from build123d import *

# Parameters (mm, degrees)
IZIM1_W                     = 35
IZIM1_H                     = 35
IZIM1_W_2                   = 29
IZIM1_H_2                   = 29
Y_KSEKLIK_EKSTR_ZYON1_DEPTH = 35
IZIM2_W                     = 35
IZIM2_H                     = 35
Y_KSEKLIK_EKSTR_ZYON2_DEPTH = 2.5
IZIM7_R                     = 1.25
KES_EKSTR_ZYON5_DEPTH       = 75.246212025
IZIM5_R                     = 9.125
KES_EKSTR_ZYON3_DEPTH       = 72.894019223
IZIM10_W                    = 50
IZIM10_H                    = 50
IZIM10_W_2                  = 30.1
IZIM10_H_2                  = 30.1
Y_KSEKLIK_EKSTR_ZYON3_DEPTH = 75
IZIM12_W                    = 50
IZIM12_H                    = 50
IZIM12_W_2                  = 35
IZIM12_H_2                  = 35
Y_KSEKLIK_EKSTR_ZYON4_DEPTH = 20
KES_EKSTR_ZYON1_DEPTH       = 121.545634512
KES_EKSTR_ZYON6_START       = -10
KES_EKSTR_ZYON6_DEPTH       = 10
DAIRESEL_KAPLAMA1_COUNT     = 4
KES_EKSTR_ZYON7_DEPTH       = 124.389626793
KES_EKSTR_ZYON8_DEPTH       = 124.389626793
RADYUS4_R                   = 10
KES_EKSTR_ZYON9_DEPTH       = 121.545634512


with BuildPart() as part:
    # izim1 → Y_kseklik-Ekstr_zyon1 (new, symmetric)
    with BuildSketch(Plane.XY):
        Rectangle(IZIM1_W, IZIM1_H)
        Rectangle(IZIM1_W_2, IZIM1_H_2, mode=Mode.SUBTRACT)
    extrude(amount=Y_KSEKLIK_EKSTR_ZYON1_DEPTH, both=True)

    # izim2 → Y_kseklik-Ekstr_zyon2 (add)
    with BuildSketch(Plane.XY.offset(35)):
        Rectangle(IZIM2_W, IZIM2_H)
    extrude(amount=-Y_KSEKLIK_EKSTR_ZYON2_DEPTH)

    # izim7 → Kes-Ekstr_zyon5 (cut, through all)
    with BuildSketch(Plane.XY.offset(35)):
        with Locations((-11, 0)):
            Circle(IZIM7_R)
        with Locations((11, 0)):
            Circle(IZIM7_R)
        with Locations((0, 11)):
            Circle(IZIM7_R)
        with Locations((0, -11)):
            Circle(IZIM7_R)
    extrude(amount=-KES_EKSTR_ZYON5_DEPTH, mode=Mode.SUBTRACT)

    # izim5 → Kes-Ekstr_zyon3 (cut, through all)
    with BuildSketch(Plane(origin=(0, 0, 32.5), x_dir=(-1, 0, 0), z_dir=(0, 0, -1))):
        Circle(IZIM5_R)
    extrude(amount=-KES_EKSTR_ZYON3_DEPTH, mode=Mode.SUBTRACT)



with BuildPart() as body_2:
    # izim10 → Y_kseklik-Ekstr_zyon3 (new body)
    with BuildSketch(Plane(origin=(0, 0, -35), x_dir=(-1, 0, 0), z_dir=(0, 0, -1))):
        Rectangle(IZIM10_W, IZIM10_H)
        Rectangle(IZIM10_W_2, IZIM10_H_2, mode=Mode.SUBTRACT)
    extrude(amount=Y_KSEKLIK_EKSTR_ZYON3_DEPTH)


with BuildPart() as part_1:
    add(part.part)

    add(body_2.part)  # Y_kseklik-Ekstr_zyon4 merges body 2
    # izim12 → Y_kseklik-Ekstr_zyon4 (add)
    with BuildSketch(Plane.XY.offset(-35)):
        Rectangle(IZIM12_W, IZIM12_H)
        Rectangle(IZIM12_W_2, IZIM12_H_2, mode=Mode.SUBTRACT)
    extrude(amount=Y_KSEKLIK_EKSTR_ZYON4_DEPTH)

    # izim3 → Kes-Ekstr_zyon1 (cut, through all)
    with BuildSketch(Plane(origin=(0, 17.5, 0), x_dir=(1, 0, 0), z_dir=(0, 1, 0))):
        with BuildLine():
            Line((10, 20), (10, -20))
            ThreePointArc((10, -20), (0, -30), (-10, -20))
            Line((-10, -20), (-10, 20))
            ThreePointArc((-10, 20), (0, 30), (10, 20))
        make_face()
    kes_ekstr_zyon1 = extrude(amount=-KES_EKSTR_ZYON1_DEPTH, mode=Mode.SUBTRACT)

    # izim8 → Kes-Ekstr_zyon6 (cut)
    with BuildSketch(Plane.XZ.offset(17.5).offset(KES_EKSTR_ZYON6_START)):
        with BuildLine():
            Line((-10, -20), (-10, -35))
            Line((-10, -35), (10, -35))
            Line((10, -35), (10, -20))
            ThreePointArc((10, -20), (0, -30), (-10, -20))
        make_face()
    extrude(amount=KES_EKSTR_ZYON6_DEPTH, mode=Mode.SUBTRACT)

    # Dairesel Kaplama1: Kes-Ekstr_zyon1 ×4 about axis
    dairesel_kaplama1_axis = Axis((0, 0, 0), (0, 0, 1))
    for i in range(1, DAIRESEL_KAPLAMA1_COUNT):
        add(kes_ekstr_zyon1.rotate(dairesel_kaplama1_axis, i * 360 / DAIRESEL_KAPLAMA1_COUNT), mode=Mode.SUBTRACT)

    # izim13 → Kes-Ekstr_zyon7 (cut, through all)
    with BuildSketch(Plane(origin=(25, 0, 0), x_dir=(0, 0, -1), z_dir=(1, 0, 0))):
        Polygon((15, 25), (15, 17.5), (35, 25), align=None)
        Polygon((15, -17.5), (15, -25), (35, -25), align=None)
    extrude(amount=-KES_EKSTR_ZYON7_DEPTH, mode=Mode.SUBTRACT)

    # izim14 → Kes-Ekstr_zyon8 (cut, through all)
    with BuildSketch(Plane.XZ.offset(25)):
        Polygon((-17.5, -15), (-25, -35), (-25, -15), align=None)
        Polygon((17.5, -15), (25, -15), (25, -35), align=None)
    extrude(amount=-KES_EKSTR_ZYON8_DEPTH, mode=Mode.SUBTRACT)

    # Radyus4
    # the kernel refuses this fillet: 10 mm, written as the material it takes off along each edge
    with BuildSketch(Plane(origin=(32.317073171, 32.317073171, -54.512195122), x_dir=(-0.9435273723846194, 0.11632529248577513, -0.31020077996206696), z_dir=(-0.33129457822453995, -0.3312945782245377, 0.883452208598773))) as radyus4_piece_1_section:
        with BuildLine():
            CenterArc((RADYUS4_R * 0.883452208599, RADYUS4_R), RADYUS4_R, 187.08188169, 82.91811831)
            Line((-RADYUS4_R * 0.108918765444, RADYUS4_R * 0.876712328767), (0, 0))
            Line((0, 0), (RADYUS4_R * 0.883452208599, 0))
        make_face()
    radyus4_piece_1 = extrude(amount=66.811073275, mode=Mode.PRIVATE)
    radyus4_piece_1 = split(radyus4_piece_1, bisect_by=Plane(origin=(17.5, 21.25, -29.89398757), z_dir=(1, 0, 0)), keep=Keep.TOP, mode=Mode.PRIVATE)
    add(radyus4_piece_1, mode=Mode.SUBTRACT)
    with BuildSketch(Plane(origin=(32.317073171, 32.317073171, -54.512195122), x_dir=(-0.9435273723846194, 0.11632529248577513, -0.31020077996206696), z_dir=(-0.33129457822453995, -0.3312945782245377, 0.883452208598773))) as radyus4_piece_2_section:
        with BuildLine():
            CenterArc((RADYUS4_R * 0.883452208599, RADYUS4_R), RADYUS4_R, 187.08188169, 82.91811831)
            Line((-RADYUS4_R * 0.108918765444, RADYUS4_R * 0.876712328767), (0, 0))
            Line((0, 0), (RADYUS4_R * 0.883452208599, 0))
        make_face()
    radyus4_piece_2 = extrude(amount=66.811073275, mode=Mode.PRIVATE)
    radyus4_piece_2 = split(radyus4_piece_2, bisect_by=Plane(origin=(16.256655696, 17.5, -22.379324277), z_dir=(0, 1, 0)), keep=Keep.TOP, mode=Mode.PRIVATE)
    add(radyus4_piece_2, mode=Mode.SUBTRACT)
    with BuildSketch(Plane(origin=(-10.182926829, 10.182926829, 4.512195122), x_dir=(0.943527372384614, 0.11632529248577986, -0.3102007799620813), z_dir=(-0.33129457822455505, 0.3312945782245359, -0.883452208598768))) as radyus4_piece_3_section:
        with BuildLine():
            CenterArc((RADYUS4_R * 0.883452208599, RADYUS4_R), RADYUS4_R, 187.08188169, 82.91811831)
            Line((-RADYUS4_R * 0.108918765444, RADYUS4_R * 0.876712328767), (0, 0))
            Line((0, 0), (RADYUS4_R * 0.883452208599, 0))
        make_face()
    radyus4_piece_3 = extrude(amount=66.811073275, mode=Mode.PRIVATE)
    radyus4_piece_3 = split(radyus4_piece_3, bisect_by=Plane(origin=(-17.5, 13.216664443, -19.287647888), z_dir=(-1, 0, 0)), keep=Keep.TOP, mode=Mode.PRIVATE)
    add(radyus4_piece_3, mode=Mode.SUBTRACT)
    with BuildSketch(Plane(origin=(-10.182926829, 10.182926829, 4.512195122), x_dir=(0.943527372384614, 0.11632529248577986, -0.3102007799620813), z_dir=(-0.33129457822455505, 0.3312945782245359, -0.883452208598768))) as radyus4_piece_4_section:
        with BuildLine():
            CenterArc((RADYUS4_R * 0.883452208599, RADYUS4_R), RADYUS4_R, 187.08188169, 82.91811831)
            Line((-RADYUS4_R * 0.108918765444, RADYUS4_R * 0.876712328767), (0, 0))
            Line((0, 0), (RADYUS4_R * 0.883452208599, 0))
        make_face()
    radyus4_piece_4 = extrude(amount=66.811073275, mode=Mode.PRIVATE)
    radyus4_piece_4 = split(radyus4_piece_4, bisect_by=Plane(origin=(-13.216664444, 17.5, -19.287647888), z_dir=(0, 1, 0)), keep=Keep.TOP, mode=Mode.PRIVATE)
    add(radyus4_piece_4, mode=Mode.SUBTRACT)
    with BuildSketch(Plane(origin=(10.182926829, -10.182926829, 4.512195122), x_dir=(0.11632529248577561, 0.9435273723846188, -0.3102007799620686), z_dir=(0.33129457822453945, -0.3312945782245416, -0.8834522085987717))) as radyus4_piece_5_section:
        with BuildLine():
            CenterArc((RADYUS4_R * 0.883452208599, -RADYUS4_R), RADYUS4_R, 90, 82.91811831)
            Line((-RADYUS4_R * 0.108918765444, -RADYUS4_R * 0.876712328767), (0, 0))
            Line((0, 0), (RADYUS4_R * 0.883452208599, 0))
        make_face()
    radyus4_piece_5 = extrude(amount=66.811073275, mode=Mode.PRIVATE)
    radyus4_piece_5 = split(radyus4_piece_5, bisect_by=Plane(origin=(13.216664443, -17.5, -19.287647888), z_dir=(0, -1, 0)), keep=Keep.TOP, mode=Mode.PRIVATE)
    add(radyus4_piece_5, mode=Mode.SUBTRACT)
    with BuildSketch(Plane(origin=(10.182926829, -10.182926829, 4.512195122), x_dir=(0.11632529248577561, 0.9435273723846188, -0.3102007799620686), z_dir=(0.33129457822453945, -0.3312945782245416, -0.8834522085987717))) as radyus4_piece_6_section:
        with BuildLine():
            CenterArc((RADYUS4_R * 0.883452208599, -RADYUS4_R), RADYUS4_R, 90, 82.91811831)
            Line((-RADYUS4_R * 0.108918765444, -RADYUS4_R * 0.876712328767), (0, 0))
            Line((0, 0), (RADYUS4_R * 0.883452208599, 0))
        make_face()
    radyus4_piece_6 = extrude(amount=66.811073275, mode=Mode.PRIVATE)
    radyus4_piece_6 = split(radyus4_piece_6, bisect_by=Plane(origin=(17.5, -13.216664444, -19.287647888), z_dir=(1, 0, 0)), keep=Keep.TOP, mode=Mode.PRIVATE)
    add(radyus4_piece_6, mode=Mode.SUBTRACT)
    with BuildSketch(Plane(origin=(-32.317073171, -32.317073171, -54.512195122), x_dir=(-0.11632529248578077, 0.9435273723846194, -0.31020077996206435), z_dir=(0.33129457822455455, 0.33129457822453956, 0.8834522085987668))) as radyus4_piece_7_section:
        with BuildLine():
            CenterArc((RADYUS4_R * 0.883452208599, -RADYUS4_R), RADYUS4_R, 90, 82.91811831)
            Line((-RADYUS4_R * 0.108918765444, -RADYUS4_R * 0.876712328767), (0, 0))
            Line((0, 0), (RADYUS4_R * 0.883452208599, 0))
        make_face()
    radyus4_piece_7 = extrude(amount=66.811073275, mode=Mode.PRIVATE)
    radyus4_piece_7 = split(radyus4_piece_7, bisect_by=Plane(origin=(-21.25, -17.5, -29.89398757), z_dir=(0, -1, 0)), keep=Keep.TOP, mode=Mode.PRIVATE)
    add(radyus4_piece_7, mode=Mode.SUBTRACT)
    with BuildSketch(Plane(origin=(-32.317073171, -32.317073171, -54.512195122), x_dir=(-0.11632529248578077, 0.9435273723846194, -0.31020077996206435), z_dir=(0.33129457822455455, 0.33129457822453956, 0.8834522085987668))) as radyus4_piece_8_section:
        with BuildLine():
            CenterArc((RADYUS4_R * 0.883452208599, -RADYUS4_R), RADYUS4_R, 90, 82.91811831)
            Line((-RADYUS4_R * 0.108918765444, -RADYUS4_R * 0.876712328767), (0, 0))
            Line((0, 0), (RADYUS4_R * 0.883452208599, 0))
        make_face()
    radyus4_piece_8 = extrude(amount=66.811073275, mode=Mode.PRIVATE)
    radyus4_piece_8 = split(radyus4_piece_8, bisect_by=Plane(origin=(-17.5, -16.256655696, -22.379324277), z_dir=(-1, 0, 0)), keep=Keep.TOP, mode=Mode.PRIVATE)
    add(radyus4_piece_8, mode=Mode.SUBTRACT)

    # izim15 → Kes-Ekstr_zyon9 (cut, through all)
    with BuildSketch(Plane(origin=(0, -17.5, 0), x_dir=(1, 0, 0), z_dir=(0, 1, 0))):
        with BuildLine():
            Line((10, 20), (10, 35))
            Line((10, 35), (-10, 35))
            Line((-10, 35), (-10, 20))
            ThreePointArc((-10, 20), (0, 30), (10, 20))
        make_face()
    extrude(amount=-KES_EKSTR_ZYON9_DEPTH, mode=Mode.SUBTRACT)


solid = part_1.part
Read the model definition and answer for the solid it produces. Units are mm, in the model's axes. A direction names the side the tool comes from. Coordinates: 2 decimals unless noted, no trailing zeros. Write each loop counter-clockwise with the first axis right and the second up, starting at its lowest first coordinate (ties: lowest second). Pieces come first, ordered by that corner, then holes. Notation, with made-up numbers: (-13.5, 70) -> (10.5, 70) arc R10 ccw to (10.5, 78) -> close; hole circle Ø4 at (20, -18.5). An arc over 180 degrees is marked (long way). Return JSON: item names as keys, results as strings.
(1) The part is cut by section B-B on y = -6.5. Give the vertices of the cut face in (x, z).
Answers below:
{"outline": "(-25, -110) -> (-15.05, -110) -> (-15.05, -35) -> (-14.5, -35) -> (-14.5, -27.6) -> (-22.22, -27.6) -> (-25, -35) -> close; (-17.5, 27.6) -> (-14.5, 27.6) -> (-14.5, 32.5) -> (-6.4, 32.5) -> (-6.4, 35) -> (-17.5, 35) -> close; (6.4, 32.5) -> (14.5, 32.5) -> (14.5, 27.6) -> (17.5, 27.6) -> (17.5, 35) -> (6.4, 35) -> close; (14.5, -35) -> (15.05, -35) -> (15.05, -110) -> (25, -110) -> (25, -35) -> (22.22, -27.6) -> (14.5, -27.6) -> close"}
(2) For a pull along Z with two mould halves and no side action, classify faces 4 (the flat face through (16, -10, 0)), 5 (the flat face through (8, 8, 35)), 6 (the flat face through (-15.05, 0, -72)), 7 (the flat face through (10, 16, 0)) as pulls with the +Z half, pulls with the -Z half, needs draft (parallel to the pull), parting line crosses it, or undercut.
Answers below:
{"face 4": "undercut", "face 5": "pulls with the +Z half", "face 6": "needs draft", "face 7": "undercut"}
(3) Consider line 1 along Y through (x, z) = (0, 33.1) (3 decimals); line 2 along Y through (x, z) = (-4, -57). Determine where each line is inside the solid, lowest interval first. Write a range as from..to.
Answers below:
{"line 1": "-17.5..-12.25, -9.75..-9.125, 9.125..9.75, 12.25..17.5", "line 2": "-25..-15.05, 15.05..25"}
(4) Each of these flat-tipped pins is pushed along its axis until it touches: P1, Ø4, axis at x = 0, y = -11, coming from the -Z side; P2, Ø1.5, axis at x = 8.5, y = 19, coming from the +Z side; P3, Ø3, axis at y = -17.5, z = -2, coming from the +X side. Where does it stop, or does it pass through?
Answers below:
{"P1": "z = 32.5", "P2": "z = -23.8", "P3": "x = 17.5"}
(5) Which of the six approach directions +Z, -Z, +X, -X, +Y, -Y give full straight-line access (tool end or side, diameter ignored) to faces 1 (the cylindrical face through (9.75, 0.05, 33.77)), 2 (the flat face through (-11, -14.5, 1)), 3 (the cylindrical face through (0, -16, 30))?
Answers below:
{"face 1": "+Z, -Z", "face 2": "-Z", "face 3": "+Y, -Y"}
(6) The part is cut by section A-A on z = -81. Give the vertices of the cut face in (x, y).
Answers below:
{"outline": "(-25, -25) -> (25, -25) -> (25, 25) -> (-25, 25) -> close; hole (-15.05, -15.05) -> (15.05, -15.05) -> (15.05, 15.05) -> (-15.05, 15.05) -> close"}
